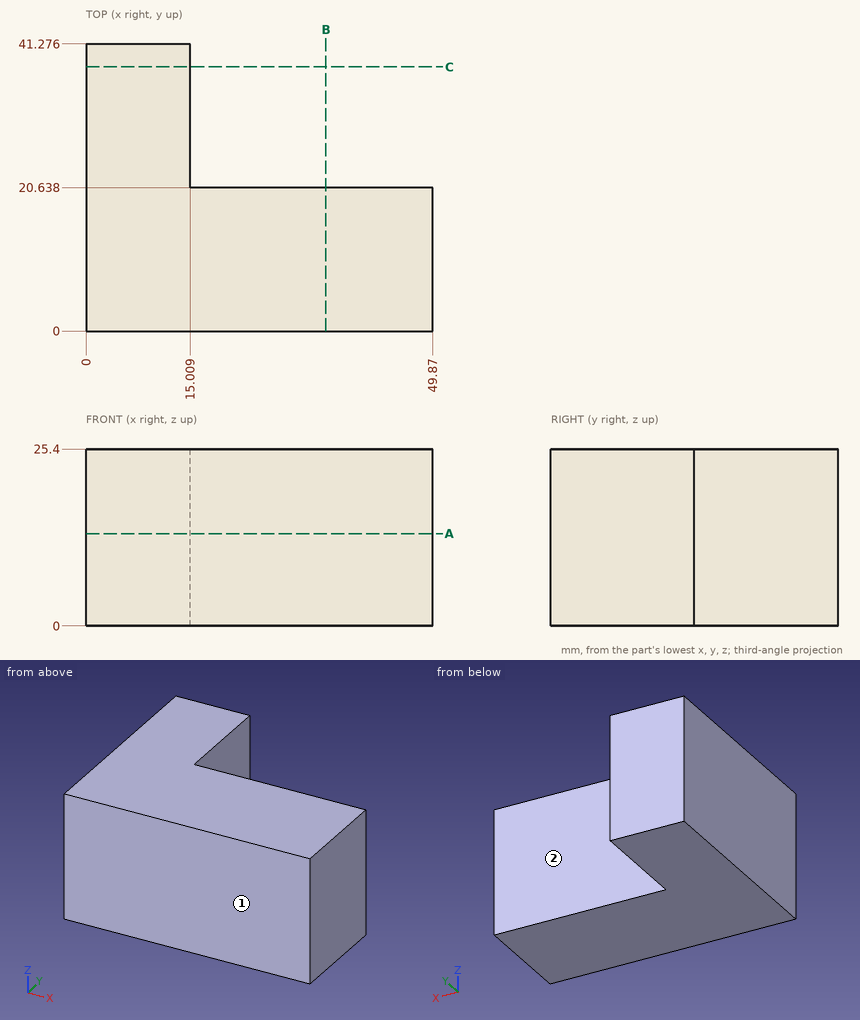
Verification items for this drawing (mm, ordinates from the low corner). A direction names the side the tool comes from. Coordinates: 2 decimals unless noted, no trailing zeros. Order: outer loops, then holes, each group sorted by start corner. A loop starts at its lowest first (then second) coordinate and runs counter-clockwise, first axis right, second up. Notation, with made-up numbers: M -33,-10.75 L 10,-10.75 A12 ccw 10,1.25 Z; hole C 22,-24 d3. An arc over 180 degrees is marked long. One line per item, written item: value. Start each with the question number.
Item 1: Sectioned sample at A-A on z = 13.25. Record the cut outline in (x, y).
Item 2: Depth check by flat-ended pin: P1, Ø7.5, axis at x = 30, z = 11, coming from the +Y side; P2, Ø2, axis at x = 15.5, z = 10.5, coming from the -Y side; P3, Ø10.5, axis at y = 31.5, z = 16.5, coming from the +X side. Enter the tip coordinate at first touch or a pass-through.
Item 3: Access from +Z, -Z, +X, -X, +Y, -Y to the whole of each face (thin tool, end or side, straight path). Record for the marked faces 1 and 2.
Item 4: Sectioned sample at B-B on x = 34.5. Record the cut outline in (y, z).
Item 5: Sectioned sample at C-C on y = 38. Record the cut outline in (x, z), then the cut area to 3 significant figures.
Item 6: Thickness scan on probe 1 along X at (y, z) = (25.5, 19.5); probe 2 along Y at (x, z) = (17.5, 7.75). Record the ranges inside material, lowest first.
Calculated:
1. outline: M 0,0 L 49.87,0 L 49.87,20.64 L 15.01,20.64 L 15.01,41.28 L 0,41.28 Z
2. P1: y = 20.64
2. P2: y = 0
2. P3: x = 15.01
3. face 1: +Z, -Z, +X, -X, -Y
3. face 2: +Z, -Z, +X, +Y
4. outline: M 0,0 L 20.64,0 L 20.64,25.4 L 0,25.4 Z
5. outline: M 0,0 L 15.01,0 L 15.01,25.4 L 0,25.4 Z
5. area: 381 mm^2
6. probe 1: 0 to 15.01
6. probe 2: 0 to 20.64
